CAD build for the part. Positions are in the model's coordinates, mm. A direction names the side the tool comes from. Coordinates: 2 decimals unless noted, no trailing zeros. Write each loop counter-clockwise with the first axis right and the second up, starting at its lowest first coordinate (ties: lowest second). Pieces come first, ordered by that corner, then holes. Notation, with made-up numbers: (19, 24) - (53, 24) arc R24 cw to (53, 52) - close; hole circle Ø8 at (70, -27.75). An arc over 180 degrees is marked (long way). Answer in a Markdown table with one row per item. Add a question column.
Q1. Band-saw the part on C-C (x = -68). List the corners of the cut face in (y, z).
Q2. Two-plate mould, pull along Z, no slides. Class faces 1 (the cylindrical face through (209.45, 69.31, -15.39)), 2 (the flat face through (-225, 27.4, -66.3)), 3 (the cylindrical face through (3.15, 66.538, 34.608)): +Z half, -Z half, draft (parallel to the pull), parting line (faces both ways), or undercut.
Q3. Band-saw the part on A-A (y = 0). List the corners of the cut face in (x, z), and give its area (3 significant figures).
Q4. Drill centre lines: line 1 along Y through (x, z) = (206, 0); line 2 along Z through (x, y) = (0, -55.5); line 3 along Y through (x, z) = (160.5, -6). Where is each one in solid material? Low to high. Write a range as from..to.
Q5. Pin check, flat tips, straight feed: pin 1 (10 mm diameter, centred on x = -22.5, z = 28.5, fed in from -Y); pin 2 (10 mm diameter, centred on x = -41.5, z = -7.5, fed in from -Y); pin 3 (4 mm diameter, centred on x = -48, y = -25.5, fed in from -Z). Stop position of each tip, or through.
Q6. 3-axis set-ups, long thin cutter, end or side, ignore diameter. For faces 4 (the cylindrical face through (2.73, 68.335, -15.175)), 5 (the flat face through (195, 47, -52.3)), 6 (the flat face through (-195, 47, -52.3)): which of +Z, -Z, +X, -X, +Y, -Y reach the whole face in a straight line?
```python
from build123d import *

# Parameters (mm, degrees)
SKETCH_1_W = 450
SKETCH_1_H = 5


with BuildPart() as part:
    # ｽｹｯﾁ1 → Revolve 585 (revolve)
    with BuildSketch(Plane.XY, mode=Mode.PRIVATE) as revolve_585_sk:
        with Locations((0, 72.5)):
            Rectangle(SKETCH_1_W, SKETCH_1_H)
    revolve(revolve_585_sk.sketch.rotate(Axis((0, 0, 0), (1, 0, 0)), 90), axis=Axis((0, 0, 0), (1, 0, 0)))

    # ｽｹｯﾁ2 → Cut-Revolve 639 (revolve, cut)
    with BuildSketch(Plane.XY, mode=Mode.PRIVATE) as cut_revolve_639_sk:
        Polygon((195, 70), (195, 71), (223.5, 71), (225, 71.55), (225, 70), align=None)
    cut_revolve_639 = revolve(cut_revolve_639_sk.sketch.rotate(Axis((0, 0, 0), (1, 0, 0)), 90), axis=Axis((0, 0, 0), (1, 0, 0)), mode=Mode.SUBTRACT)

    # Mirror 681: Cut-Revolve 639 across plane
    add(cut_revolve_639.mirror(Plane(origin=(0, 0, 0), x_dir=(0, 0, 1), z_dir=(1, 0, 0))), mode=Mode.SUBTRACT)


solid = part.part
```
Checked values:
| question | item | result |
|---|---|---|
| 1 | outline | circle Ø150 at (0, 0); hole circle Ø140 at (0, 0) |
| 2 | face 1 | undercut |
| 2 | face 2 | draft |
| 2 | face 3 | parting line |
| 3 | outline | (-225, -75) - (225, -75) - (225, -71.55) - (223.5, -71) - (195, -71) - (195, -70) - (-195, -70) - (-195, -71) - (-223.5, -71) - (-225, -71.55) - close; (-225, 71.55) - (-223.5, 71) - (-195, 71) - (-195, 70) - (195, 70) - (195, 71) - (223.5, 71) - (225, 71.55) - (225, 75) - (-225, 75) - close |
| 3 | area | 4,380 mm² |
| 4 | line 1 | y = -75..-71, 71..75 |
| 4 | line 2 | z = -50.45..-42.66, 42.66..50.45 |
| 4 | line 3 | y = -74.76..-69.74, 69.74..74.76 |
| 5 | pin 1 | stops at y = -71.22 |
| 5 | pin 2 | stops at y = -74.96 |
| 5 | pin 3 | stops at z = -71.22 |
| 6 | face 4 | +X, -X |
| 6 | face 5 | +X |
| 6 | face 6 | -X |
